```python
from build123d import *

# Parameters (mm, degrees)
F0_R     = 3.175
F1_DEPTH = 12.7


with BuildPart() as f1:
    # F0 (on Front) → F1 (new body)
    with BuildSketch(Plane.XZ):
        Polygon((0, 127), (0, 0), (63.5, 0), align=None)
        with Locations((12.7, 12.7)):
            Circle(F0_R, mode=Mode.SUBTRACT)
        with Locations((38.1, 12.7)):
            Circle(F0_R, mode=Mode.SUBTRACT)
    extrude(amount=F1_DEPTH)


solid = f1.part
```
For this review, take the finished solid that the model builds, in its own axes (mm). Round coordinates to 2 decimals unless told otherwise and drop trailing zeros. Order: outer loops, then holes, each group sorted by start corner. A loop starts at its lowest first (then second) coordinate and runs counter-clockwise, first axis right, second up.
Q1. Mouldability with a two-part tool opening along Z and no side actions: class faces 1 (the cylindrical face through (10.18, -6.26, 10.77)), 2 (the flat face through (32, -6, 63)), 3 (the flat face through (0, -6, 64)) as pulls with the +Z half, pulls with the -Z half, needs draft (parallel to the pull), parting line crosses it, or undercut.
Findings below:
face 1: undercut
face 2: pulls with the +Z half
face 3: needs draft
Q2. Insertion check: P1, Ø6, axis at x = 15, y = -4.5, coming from the +Z side; P2, Ø5, axis at y = -3.5, z = 19, coming from the +X side; P3, Ø1, axis at y = -6, z = 47.5, coming from the +X side. Each pin has a flat end and moves straight along its axis. Give the tip position at first contact, or say it passes through.
Findings below:
P1: stops at z = 103
P2: stops at x = 55.25
P3: stops at x = 40
Q3. We need section A-A, the plane x = 12.7. Give the boundary of the cut face in (y, z) (3 decimals).
Findings below:
outline: (-12.7, 0) - (0, 0) - (0, 9.525) - (-12.7, 9.525) - close; (-12.7, 15.875) - (0, 15.875) - (0, 101.6) - (-12.7, 101.6) - close
Q4. Wall thickness on line 1 (Z direction, x = 12.7, y = -8.25) (3 decimals); line 2 (Z direction, x = 38.1, y = -4.25) (3 decimals); line 3 (Z direction, x = 22.5, y = -3.75): over which ranges is each line inside the solid? List them lowest first.
Findings below:
line 1: z = 0 to 9.525, 15.875 to 101.6
line 2: z = 0 to 9.525, 15.875 to 50.8
line 3: z = 0 to 82
Q5. We need section D-D, the plane x = 38.1. Give the boundary of the cut face in (y, z) (3 decimals), plus the area to 3 significant figures.
Findings below:
outline: (-12.7, 0) - (0, 0) - (0, 9.525) - (-12.7, 9.525) - close; (-12.7, 15.875) - (0, 15.875) - (0, 50.8) - (-12.7, 50.8) - close
area: 565 mm2
Q6. We need section B-B, the plane z = 12.7. Give the boundary of the cut face in (x, y) (3 decimals).
Findings below:
outline: (0, -12.7) - (9.525, -12.7) - (9.525, 0) - (0, 0) - close; (15.875, -12.7) - (34.925, -12.7) - (34.925, 0) - (15.875, 0) - close; (41.275, -12.7) - (57.15, -12.7) - (57.15, 0) - (41.275, 0) - close
Q7. We need section C-C, the plane y = -9. Give the boundary of the cut face in (x, z) (3 decimals).
Findings below:
outline: (0, 0) - (63.5, 0) - (0, 127) - close; hole circle Ø6.35 at (12.7, 12.7); hole circle Ø6.35 at (38.1, 12.7)
